Build history of the part. All positions in model axes, mm. A direction names the side the tool comes from. Coordinates: 2 decimals unless noted, no trailing zeros. Loops run counter-clockwise (first coordinate to the right, second up) from the corner with the lowest first, then second, coordinate; pieces in that order, holes last.
Item 1: Cut at D-D (z = -76.5). List the corners of the cut face in (x, y), and give its area (3 significant figures).
Item 2: Cut at A-A (y = -46.5). List the corners of the cut face in (x, z), and give its area (3 significant figures).
Item 3: Mould opens along Z. For faces 1 (the face through (33, -42.1, -102)), 2 (the face through (33, -29, -32)), 3 (the face through (33, 1, -93.644)) say: released by +Z, released by -Z, zero draft, split by the parting line, or undercut.
Item 4: Drill centre lines: line 1 along Z through (x, y) = (33.35, -58); line 2 along Z through (x, y) = (33.85, -37.5); line 3 along Z through (x, y) = (34.6, -31). Where is each one in solid material? Low to high.
Item 5: Cut at B-B (y = -20.5). List the corners of the cut face in (x, z), and give its area (3 significant figures).
Item 6: Cut at C-C (z = -7.5). List the corners of the cut face in (x, y), and give its area (3 significant figures).
Item 7: 3-axis set-ups, long thin cutter, end or side, ignore diameter. For faces 4 (the face through (33, -31.9, -102)), 5 (the face through (33, -66.9, 34)), 6 (the face through (33, -51, -13)), 7 (the face through (33, -57, 31)), 8 (the face through (33, -22.1, -19)): which of +Z, -Z, +X, -X, +Y, -Y reach the whole face in a straight line?
Item 8: Flat gauge pins, fed straight in: pin 1 (1.5 mm diameter, centred on x = 33.5, z = 34, fed in from -Y); pin 2 (1.5 mm diameter, centred on x = 32.5, y = 0, fed in from -Z); pin 3 (1 mm diameter, centred on x = 34, z = -62.5, fed in from +Y). Where does each tip first touch, or does it go through?
from build123d import *

# Parameters (mm, degrees)
BOSS_EXTRUDE1_DEPTH = 3
SKETCH6_W           = 3.2
SKETCH6_H           = 10.2
SKETCH6_H_2         = 5.2
SKETCH6_W_2         = 10.2
SKETCH6_H_3         = 3.2
CUT_EXTRUDE1_DEPTH  = 4
BOSS_EXTRUDE2_DEPTH = 3


with BuildPart() as part:
    # Sketch2 → Boss-Extrude1 (new body)
    with BuildSketch(Plane(origin=(34.872217102, 0, 0), x_dir=(0, 0, -1), z_dir=(1, 0, 0))):
        Polygon((103.744434203, 3), (103.744434203, -72), (-35.95, -72), (-35.95, -57), (17, -57), (17, 3), (32, 3), (32, -57), (88.744434203, -57), (88.744434203, 3), align=None)
    extrude(amount=-BOSS_EXTRUDE1_DEPTH)

    # Sketch6 → Cut-Extrude1 (cut, through all)
    with BuildSketch(Plane(origin=(34.872217102, 0, 0), x_dir=(0, 0, -1), z_dir=(1, 0, 0))):
        with Locations((102.244434203, -37)):
            Rectangle(SKETCH6_W, SKETCH6_H)
        with Locations((102.244434203, -57)):
            Rectangle(SKETCH6_W, SKETCH6_H)
        with Locations((102.244434203, -17)):
            Rectangle(SKETCH6_W, SKETCH6_H)
        with Locations((-34.45, -69.5)):
            Rectangle(SKETCH6_W, SKETCH6_H_2)
        with Locations((-20.95, -58.5)):
            Rectangle(SKETCH6_W_2, SKETCH6_H_3)
        with Locations((39.05, -58.5)):
            Rectangle(SKETCH6_W_2, SKETCH6_H_3)
        with Locations((-0.95, -58.5)):
            Rectangle(SKETCH6_W_2, SKETCH6_H_3)
        with Locations((18.5, -17)):
            Rectangle(SKETCH6_W, SKETCH6_H)
        with Locations((79.05, -58.5)):
            Rectangle(SKETCH6_W_2, SKETCH6_H_3)
        with Locations((59.05, -58.5)):
            Rectangle(SKETCH6_W_2, SKETCH6_H_3)
        Polygon((16.9, 2.4), (21.9, 2.4), (21.9, -0.85), (32.1, -0.85), (32.1, 3.1), (16.9, 3.1), align=None)
        Polygon((93.644434203, -0.85), (100.644434203, -0.85), (100.644434203, -2.1), (103.844434203, -2.1), (103.844434203, 3.1), (88.644434203, 3.1), (88.644434203, 2.4), (93.644434203, 2.4), align=None)
        with Locations((18.5, -37)):
            Rectangle(SKETCH6_W, SKETCH6_H)
    extrude(amount=-CUT_EXTRUDE1_DEPTH, mode=Mode.SUBTRACT)

    # Sketch8 → Boss-Extrude2 (add)
    with BuildSketch(Plane(origin=(34.872217102, 0, 0), x_dir=(0, 0, -1), z_dir=(1, 0, 0))):
        Polygon((13, -53), (13, -49), (5, -49), (5, -57), (9, -57), (9, -53), align=None)
    extrude(amount=-BOSS_EXTRUDE2_DEPTH)


solid = part.part
Filled sheet:
1. outline: (31.87, -72) - (34.87, -72) - (34.87, -60.1) - (31.87, -60.1) - close
1. area: 35.7 mm2
2. outline: (31.87, -103.74) - (34.87, -103.74) - (34.87, -88.74) - (31.87, -88.74) - close; (31.87, -32) - (34.87, -32) - (34.87, -17) - (31.87, -17) - close
2. area: 90.0 mm2
3. face 1: zero draft
3. face 2: undercut
3. face 3: released by -Z
4. line 1: z = -100.64 to -84.15, -73.95 to -64.15, -53.95 to -44.15, -33.95 to -4.15, 6.05 to 15.85, 26.05 to 35.95
4. line 2: z = -100.64 to -88.74, -32 to -20.1
4. line 3: z = -103.74 to -88.74, -32 to -17
5. outline: (31.87, -100.64) - (34.87, -100.64) - (34.87, -88.74) - (31.87, -88.74) - close; (31.87, -32) - (34.87, -32) - (34.87, -20.1) - (31.87, -20.1) - close
5. area: 71.4 mm2
6. outline: (31.87, -72) - (34.87, -72) - (34.87, -49) - (31.87, -49) - close
6. area: 69.0 mm2
7. face 4: -Z, +X, -X
7. face 5: +Z, +X, -X, -Y
7. face 6: +X, -X, +Y
7. face 7: +Z, +X, -X, +Y
7. face 8: +Z, +X, -X
8. pin 1: stops at y = -66.9
8. pin 2: stops at z = -93.64
8. pin 3: stops at y = -60.1
